Verification items for the finished model (mm, model axes). A direction names the side the tool comes from. Coordinates: 2 decimals unless noted, no trailing zeros. Write each loop counter-clockwise with the first axis right and the second up, starting at its lowest first coordinate (ties: lowest second). Pieces come first, ordered by that corner, then holes. Notation, with made-up numbers: (21, -13.75) -> (67, -13.75) arc R13 cw to (67, 1.25) -> close; hole circle Ø8 at (48.25, 23.5). An arc over 180 degrees is marked (long way). Write item = value, one per line. Start each with the question number.
(1) Section check C-C (x = 30). Record the cut outline in (y, z), plus the area to 3 significant figures.
(2) Gauge pin test, flat ends, axial feed: pin 1 Ø8 at (y, z) = (507.5, 8.5) entering from -X; pin 2 Ø2 at (y, z) = (471, 25.5) entering from +X. Record the tip position at first contact, or that the pin passes through.
(3) Set-up check for faces 4 (the face through (50, 385, -1)), 5 (the face through (1, 790, 13)), 6 (the face through (1, 385, 50)), 7 (the face through (-50, 385, 1)), 8 (the face through (-1, 0, 1)): record each of +Z, -Z, +X, -X, +Y, -Y from which the full face is reachable in a straight line by a thin tool's end or side.
(4) Section check B-B (z = 33). Record the cut outline in (x, y), plus the area to 3 significant figures.
(5) Section check A-A (y = 108). Record the cut outline in (x, z), plus the area to 3 significant figures.
(6) Mould release check, pull along Y, two halves, no side actions. Record for faces 1 (the face through (1, 385, -47)), 2 (the face through (1, 396, -50)), 3 (the face through (-1, -10, 13)): released by +Y, released by -Y, zero draft, split by the parting line, or undercut.
(7) Material ranges on probe 1 along Z at (x, y) = (-62, 782); probe 2 along X at (y, z) = (786, -37); probe 3 along X at (y, z) = (755, -31), recorded low to high. Write a range as [from, to].
```python
from build123d import *

# Parameters (mm, degrees)
F1_DEPTH = 780
F3_W     = 150
F3_H     = 125
F3_R     = 6
F4_DEPTH = 10
F7_W     = 150
F7_H     = 125
F7_R     = 6
F8_DEPTH = 10


with BuildPart() as f1:
    # F0 (on Front) → F1 (new body)
    with BuildSketch(Plane.XZ):
        with BuildLine():
            ThreePointArc((50, 45), (48.5355339059, 48.5355339059), (45, 50))
            Line((45, 50), (-45, 50))
            ThreePointArc((-45, 50), (-48.5355339059, 48.5355339059), (-50, 45))
            Line((-50, 45), (-50, -45))
            ThreePointArc((-50, -45), (-48.5355339059, -48.5355339059), (-45, -50))
            Line((-45, -50), (45, -50))
            ThreePointArc((45, -50), (48.5355339059, -48.5355339059), (50, -45))
            Line((50, -45), (50, 45))
        make_face()
        with BuildLine():
            ThreePointArc((-47, 45), (-46.4142135624, 46.4142135624), (-45, 47))
            Line((-45, 47), (45, 47))
            ThreePointArc((45, 47), (46.4142135624, 46.4142135624), (47, 45))
            Line((47, 45), (47, -45))
            ThreePointArc((47, -45), (46.4142135624, -46.4142135624), (45, -47))
            Line((45, -47), (-45, -47))
            ThreePointArc((-45, -47), (-46.4142135624, -46.4142135624), (-47, -45))
            Line((-47, -45), (-47, 45))
        make_face(mode=Mode.SUBTRACT)
    extrude(amount=-F1_DEPTH)


with BuildPart() as f4:
    # F3 (on offset) → F4 (new body)
    with BuildSketch(Plane.XZ.offset(10)):
        with Locations((0, 12.5)):
            Rectangle(F3_W, F3_H)
        with Locations((-62.5, -37.5)):
            Circle(F3_R, mode=Mode.SUBTRACT)
        with Locations((-62.5, 7.5)):
            Circle(F3_R, mode=Mode.SUBTRACT)
        with Locations((62.5, -37.5)):
            Circle(F3_R, mode=Mode.SUBTRACT)
        with Locations((62.5, 7.5)):
            Circle(F3_R, mode=Mode.SUBTRACT)
        with Locations((-62.5, 62.5)):
            Circle(F3_R, mode=Mode.SUBTRACT)
        with Locations((0, 62.5)):
            Circle(F3_R, mode=Mode.SUBTRACT)
        with Locations((62.5, 62.5)):
            Circle(F3_R, mode=Mode.SUBTRACT)
    extrude(amount=-F4_DEPTH)


with BuildPart() as f1_1:
    add(f1.part)

    # F5: union F4
    add(f4.part)

    # F7 (on offset) → F8 (join)
    with BuildSketch(Plane(origin=(0, 790, 0), x_dir=(-1, 0, 0), z_dir=(0, 1, 0))):
        with Locations((0, 12.5)):
            Rectangle(F7_W, F7_H)
        with Locations((-62.5, -37.5)):
            Circle(F7_R, mode=Mode.SUBTRACT)
        with Locations((-62.5, 7.5)):
            Circle(F7_R, mode=Mode.SUBTRACT)
        with Locations((62.5, -37.5)):
            Circle(F7_R, mode=Mode.SUBTRACT)
        with Locations((62.5, 7.5)):
            Circle(F7_R, mode=Mode.SUBTRACT)
        with Locations((-62.5, 62.5)):
            Circle(F7_R, mode=Mode.SUBTRACT)
        with Locations((0, 62.5)):
            Circle(F7_R, mode=Mode.SUBTRACT)
        with Locations((62.5, 62.5)):
            Circle(F7_R, mode=Mode.SUBTRACT)
    extrude(amount=-F8_DEPTH)


solid = f1_1.part
```
Response:
q1.outline = (-10, -50) -> (790, -50) -> (790, 75) -> (780, 75) -> (780, 50) -> (0, 50) -> (0, 75) -> (-10, 75) -> close; hole (0, -47) -> (780, -47) -> (780, 47) -> (0, 47) -> close
q1.area = 7,180 mm2
q2.pin_1 = -50
q2.pin_2 = 50
q3.face_4 = +Z, -Z, +X
q3.face_5 = +Z, -Z, +X, -X, +Y
q3.face_6 = +Z, +X, -X
q3.face_7 = +Z, -Z, -X
q3.face_8 = none
q4.outline = (-75, -10) -> (75, -10) -> (75, 0) -> (50, 0) -> (50, 780) -> (75, 780) -> (75, 790) -> (-75, 790) -> (-75, 780) -> (-50, 780) -> (-50, 0) -> (-75, 0) -> close; hole (-47, 0) -> (47, 0) -> (47, 780) -> (-47, 780) -> close
q4.area = 7,680 mm2
q5.outline = (-50, -45) arc R5 ccw to (-45, -50) -> (45, -50) arc R5 ccw to (50, -45) -> (50, 45) arc R5 ccw to (45, 50) -> (-45, 50) arc R5 ccw to (-50, 45) -> close; hole (-47, -45) arc R2 ccw to (-45, -47) -> (45, -47) arc R2 ccw to (47, -45) -> (47, 45) arc R2 ccw to (45, 47) -> (-45, 47) arc R2 ccw to (-47, 45) -> close
q5.area = 1,150 mm2
q6.face_1 = undercut
q6.face_2 = zero draft
q6.face_3 = released by -Y
q7.probe_1 = [-50, -43.48], [-31.52, 1.52], [13.48, 56.52], [68.48, 75]
q7.probe_2 = [-75, -68.48], [-56.52, 56.52], [68.48, 75]
q7.probe_3 = [-50, -47], [47, 50]
